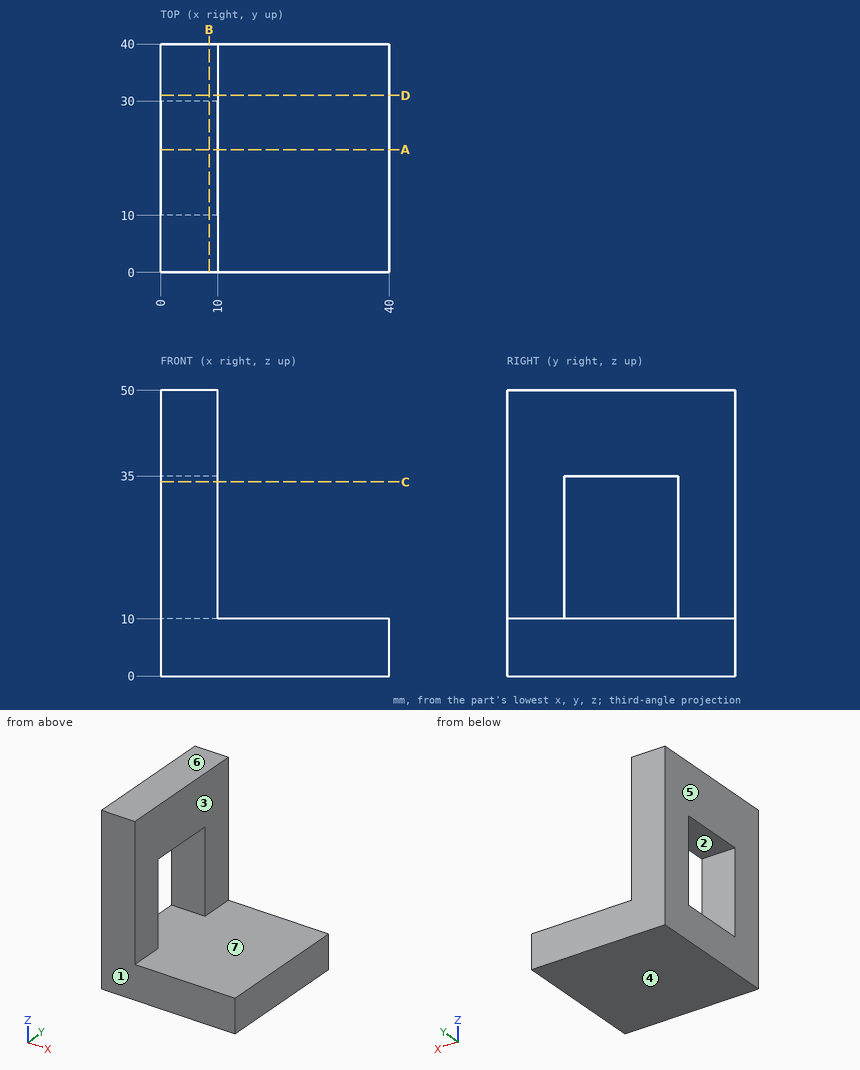
Part print with two shaded views. Sizes in mm from the minimum x, y, z corner. A direction names the side the tool comes from. Round coordinates to 2 decimals unless told otherwise and drop trailing zeros. Order: outer loops, then holes, each group sorted by start corner. A loop starts at its lowest first (then second) coordinate and runs counter-clockwise, first axis right, second up. Notation, with made-up numbers: M 25,-18.75 L 77,-18.75 A20 cw 77,1.25 Z; hole C 28,34.25 d7. An arc over 180 degrees is marked long. Answer in a Markdown table with one row per item. Add a question column.
Q1. Cut at C-C on z = 34. Give the cut face in (x, y), and give its area (3 significant figures).
Q2. Pin check, flat tip, straight feed: pin 1 (12 mm diameter, centred on x = 26.5, y = 26, fed in from +Z). Stop position of the tip, or through.
Q3. Cut at B-B on x = 8.5. Give the cut face in (y, z), and give its area (3 significant figures).
Q4. Cut at D-D on y = 31. Give the cut face in (x, z).
Q5. 3-axis set-ups, long thin cutter, end or side, ignore diameter. For the marked faces 1, 2 and 3: which of +Z, -Z, +X, -X, +Y, -Y reach the whole face in a straight line?
Q6. Cut at A-A on y = 21.5. Give the cut face in (x, z).
Q7. Wall check: L1, parallel to Z at x = 4.5, y = 25.5; L2, parallel to Y at x = 3, z = 27; L3, parallel to Z at x = 23.5, y = 19. Give the ranges that are in metal, low to high. Write a range as from..to.
Q8. Mould opens along Z. For the marked faces 4, 5, 6 and 7 say: +Z half, -Z half, draft (parallel to the pull), parting line (faces both ways), or undercut.
Established:
| question | item | result |
|---|---|---|
| 1 | outline | M 0,0 L 10,0 L 10,10 L 0,10 Z; M 0,30 L 10,30 L 10,40 L 0,40 Z |
| 1 | area | 200 mm2 |
| 2 | pin 1 | stops at z = 10 |
| 3 | outline | M 0,0 L 40,0 L 40,50 L 0,50 Z; hole M 10,10 L 30,10 L 30,35 L 10,35 Z |
| 3 | area | 1,500 mm2 |
| 4 | outline | M 0,0 L 40,0 L 40,10 L 10,10 L 10,50 L 0,50 Z |
| 5 | face 1 | +Z, -Z, +X, -X, -Y |
| 5 | face 2 | +X, -X |
| 5 | face 3 | +Z, +X, +Y, -Y |
| 6 | outline | M 0,0 L 40,0 L 40,10 L 0,10 Z; M 0,35 L 10,35 L 10,50 L 0,50 Z |
| 7 | L1 | z = 0..10, 35..50 |
| 7 | L2 | y = 0..10, 30..40 |
| 7 | L3 | z = 0..10 |
| 8 | face 4 | -Z half |
| 8 | face 5 | draft |
| 8 | face 6 | +Z half |
| 8 | face 7 | undercut |
